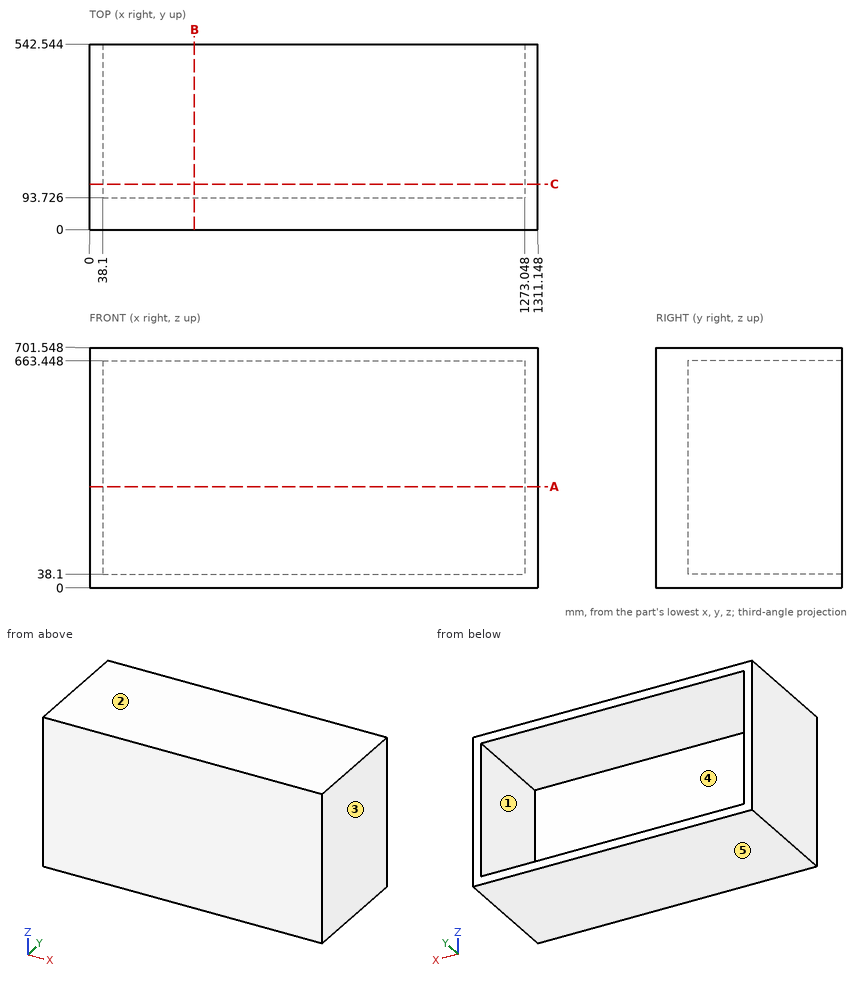
Input: dimensioned drawing with shaded views. Units: mm. Origin: part minimum x, y, z. A direction names the side the tool comes from. Coordinates: 2 decimals unless noted, no trailing zeros. Write each loop counter-clockwise with the first axis right and the second up, starting at its lowest first coordinate (ties: lowest second). Pieces come first, ordered by that corner, then holes. Notation, with made-up numbers: M -0.75,-31 L 28.25,-31 A16 cw 28.25,-7 Z; hole C 36.25,55 d9. An arc over 180 degrees is marked long. Answer as a JSON object with one key per item and string values. Group by question number.
(1) Section C-C on y = 133. Output: boundary loops of the cut face in (x, z), plus the area to 3 significant figures.
(2) Set-up query: the marked faces 1 and 2. Return all of +Z, -Z, +X, -X, +Y, -Y with unobstructed straight access to the full face (end or side cutting, diameter ignored); none if empty.
(3) Ray query, line 1 along Z through (x, y) = (628, 332); line 2 along X through (y, z) = (101, 493.5); line 3 along Y through (x, z) = (858, 404.5). Return the intervals inside material, ascending. Write a range as [from, to].
(4) Section B-B on x = 306.5. Output: boundary loops of the cut face in (y, z), plus the area to 4 significant figures.
(5) Mould query, pull axis X, two halves, no side actions, for the marked faces 3, 4 and 5. Classes: pulls with the +X half, pulls with the -X half, needs draft (parallel to the pull), parting line crosses it, or undercut.
(6) Contact query for a flat-ended pin moving along its axis: P1, Ø6, axis at x = 535, z = 525, coming from the +Y side. Output: stop coordinate, or through.
(7) Section A-A on z = 295. Output: boundary loops of the cut face in (x, y), plus the area to 3 significant figures.
Result set:
{
 "1": {"outline": "M 0,0 L 1311.15,0 L 1311.15,701.55 L 0,701.55 Z; hole M 38.1,38.1 L 1273.05,38.1 L 1273.05,663.45 L 38.1,663.45 Z", "area": "148,000 mm2"},
 "2": {"face 1": "+Y", "face 2": "+Z, +X, -X, +Y, -Y"},
 "3": {"line 1": "z = [0, 38.1], [663.45, 701.55]", "line 2": "x = [0, 38.1], [1273.05, 1311.15]", "line 3": "y = [0, 93.73]"},
 "4": {"outline": "M 0,0 L 542.54,0 L 542.54,38.1 L 93.73,38.1 L 93.73,663.45 L 542.54,663.45 L 542.54,701.55 L 0,701.55 Z", "area": "100,000 mm2"},
 "5": {"face 3": "pulls with the +X half", "face 4": "undercut", "face 5": "needs draft"},
 "6": {"P1": "stops at y = 93.73"},
 "7": {"outline": "M 0,0 L 1311.15,0 L 1311.15,542.54 L 1273.05,542.54 L 1273.05,93.73 L 38.1,93.73 L 38.1,542.54 L 0,542.54 Z", "area": "157,000 mm2"}
}
